```python
from build123d import *

# Parameters (mm, degrees)
SKETCH1_W           = 33
SKETCH1_H           = 10
BOSS_EXTRUDE1_DEPTH = 1
SKETCH3_W           = 5
SKETCH3_H           = 5
BOSS_EXTRUDE2_DEPTH = 1.2
LPATTERN1_COUNT     = 13
LPATTERN1_PITCH     = 33
LPATTERN1_COL_COUNT = 13
LPATTERN1_COL_PITCH = 33


with BuildPart() as part:
    # Sketch1 → Boss-Extrude1 (new body)
    with BuildSketch(Plane(origin=(0, 0, 0), x_dir=(1, 0, 0), z_dir=(0, 1, 0))):
        Rectangle(SKETCH1_W, SKETCH1_H)
    boss_extrude1 = extrude(amount=BOSS_EXTRUDE1_DEPTH)

    # Sketch3 → Boss-Extrude2 (add)
    with BuildSketch(Plane(origin=(0, 1, 0), x_dir=(1, 0, 0), z_dir=(0, 1, 0))):
        Rectangle(SKETCH3_W, SKETCH3_H)
    boss_extrude2 = extrude(amount=BOSS_EXTRUDE2_DEPTH)

    # LPattern1: Boss-Extrude1, Boss-Extrude2 ×13
    with Locations(*[(-i * LPATTERN1_PITCH, 0, 0) for i in range(1, LPATTERN1_COUNT)]):
        add(boss_extrude1)
        add(boss_extrude2)

    # LPattern1 col: Boss-Extrude1, Boss-Extrude2 ×13
    with Locations(*[(i * LPATTERN1_COL_PITCH, 0, 0) for i in range(1, LPATTERN1_COL_COUNT)]):
        add(boss_extrude1)
        add(boss_extrude2)


solid = part.part
```
CAD build for the part. Positions are in the model's coordinates, mm. Round coordinates to 2 decimals unless told otherwise and drop trailing zeros. Order: outer loops, then holes, each group sorted by start corner. A loop starts at its lowest first (then second) coordinate and runs counter-clockwise, first axis right, second up. Notation, with made-up numbers: (24.25, -29) - (79.25, -29) arc R16 ccw to (79.25, -15) - close; hole circle Ø2 at (83, 43.5). An arc over 180 degrees is marked (long way). Answer in a Markdown table with one row per item. Add a question column.
(1) Band-saw the part on B-B on x = -244. List the corners of the cut face in (y, z), and give its area (3 significant figures).
(2) Drop flat-ended pins along their axis: pin 1 Ø1 at (y, z) = (2, -1) entering from -X; pin 2 Ø3 at (x, z) = (185, 2.5) entering from +Y; pin 3 Ø1.5 at (x, z) = (-204.5, 4) entering from -Y; pin 4 Ø0.6 at (y, z) = (1.5, -1) entering from +X. Give the stop position or say it passes through.
(3) Probe L1, parallel to Z at x = -35, y = 1.4; L2, parallel to Y at x = 241, z = -0.25. List the from-to ranges inside material, lowest first. Write a range as [from, to].
(4) Band-saw the part on A-A on y = 1.4. Count the separate pieces of the cut face and the enclosed holes in it, and give its area (3 significant figures).
Data:
| question | item | result |
|---|---|---|
| 1 | outline | (0, -5) - (1, -5) - (1, 5) - (0, 5) - close |
| 1 | area | 10.0 mm^2 |
| 2 | pin 1 | stops at x = -398.5 |
| 2 | pin 2 | stops at y = 1 |
| 2 | pin 3 | stops at y = 0 |
| 2 | pin 4 | stops at x = 398.5 |
| 3 | L1 | z = [-2.5, 2.5] |
| 3 | L2 | y = [0, 1] |
| 4 | separate pieces | 25 |
| 4 | enclosed holes | 0 |
| 4 | area | 625 mm^2 |
